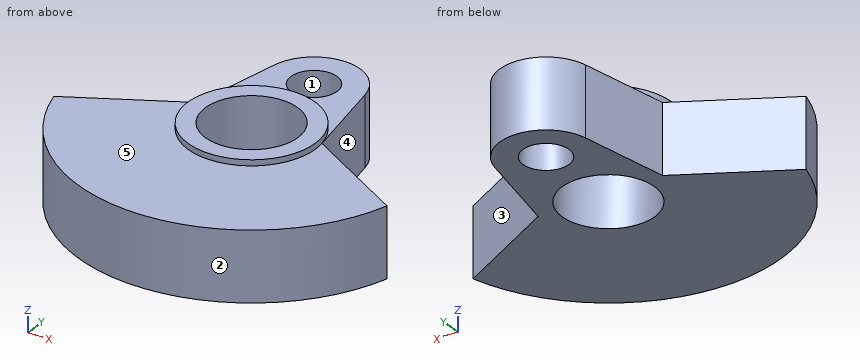
```python
from build123d import *

# Parameters (mm, degrees)
SKETCH1_R           = 2
SKETCH1_R_2         = 4
BOSS_EXTRUDE1_DEPTH = 6
SKETCH2_R           = 5.5
BOSS_EXTRUDE2_DEPTH = 0.5
CUT_EXTRUDE1_START  = -10.5
SKETCH3_R           = 4
CUT_EXTRUDE1_DEPTH  = 10.5


with BuildPart() as part:
    # Sketch1 → Boss-Extrude1 (new body)
    with BuildSketch(Plane.XY):
        with BuildLine():
            Line((-5.402455316, -6.96875), (-3.929058411, 0.75))
            ThreePointArc((-3.929058411, 0.75), (0, 4), (3.929058411, 0.75))
            Line((3.929058411, 0.75), (5.402455316, -6.96875))
            Line((5.402455316, -6.96875), (14.456832295, -12))
            ThreePointArc((14.456832295, -12), (0, -23), (-14.456832295, -12))
            Line((-14.456832295, -12), (-5.402455316, -6.96875))
        make_face()
        Circle(SKETCH1_R, mode=Mode.SUBTRACT)
        with Locations((0, -8)):
            Circle(SKETCH1_R_2, mode=Mode.SUBTRACT)
    extrude(amount=BOSS_EXTRUDE1_DEPTH)

    # Sketch2 → Boss-Extrude2 (add)
    with BuildSketch(Plane.XY.offset(6)):
        with Locations(Location((0, -8, 0), (0, 0, 169.193077125))):
            Circle(SKETCH2_R)
    extrude(amount=BOSS_EXTRUDE2_DEPTH)

    # Sketch3 → Cut-Extrude1 (cut)
    with BuildSketch(Plane.XY.offset(6.5).offset(CUT_EXTRUDE1_START)):
        with Locations((0, -8)):
            Circle(SKETCH3_R)
    extrude(amount=CUT_EXTRUDE1_DEPTH, mode=Mode.SUBTRACT)


solid = part.part
```
Check sheet for the modelled part. Datum: model origin and axes. Units: mm. Face numbers are marked on the shaded views. A direction names the side the tool comes from. Give positions to 0.01 mm unless a question says otherwise; leave off trailing zeros. Order: outer loops, then holes, each group sorted by start corner. A loop starts at its lowest first (then second) coordinate and runs counter-clockwise, first axis right, second up. Notation, with made-up numbers: M 55.5,-14.75 L 75.5,-14.75 A9 ccw 75.5,-6.75 Z; hole C -2,22 d8. An arc over 180 degrees is marked long. Answer in a Markdown table with one row per item.
1) Cross-section at C-C, the plane y = -0.5. Enter the section's corners in (x, z).
Filled sheet:
| item | result |
|---|---|
| outline | M -4.17,0 L -1.94,0 L -1.94,6 L -4.17,6 Z; M 1.94,0 L 4.17,0 L 4.17,6 L 1.94,6 Z |
2) Cross-section at A-A, the plane z = 5. Enter the section's corners in (x, y), plus the area to 3 significant figures.
Filled sheet:
| item | result |
|---|---|
| outline | M -14.46,-12 A15 ccw 14.46,-12 L 5.4,-6.97 L 3.93,0.75 A4 ccw -3.93,0.75 L -5.4,-6.97 Z; hole C 0,-8 d8; hole C 0,0 d4 |
| area | 363 mm2 |
3) Access from +Z, -Z, +X, -X, +Y, -Y to the whole of each face (thin tool, end or side, straight path). Record for the marked faces 4 and 5.
Filled sheet:
| item | result |
|---|---|
| face 4 | +Z, -Z, +X, +Y |
| face 5 | +Z, -Y |
4) Cross-section at B-B, the plane x = 0. Enter the section's corners in (y, z), plus the area to 3 significant figures.
Filled sheet:
| item | result |
|---|---|
| outline | M -23,0 L -12,0 L -12,6.5 L -13.5,6.5 L -13.5,6 L -23,6 Z; M -4,0 L -2,0 L -2,6 L -2.5,6 L -2.5,6.5 L -4,6.5 Z; M 2,0 L 4,0 L 4,6 L 2,6 Z |
| area | 91.5 mm2 |
5) Gauge pin test, flat ends, axial feed: P1, Ø8.5, axis at x = -2, y = -1.5, coming from the +Z side; P2, Ø3, axis at x = -4, z = 3, coming from the -Y side; P3, Ø3, axis at y = -7, z = 5, coming from the +X side; P4, Ø1.5, axis at y = -20, z = 1.5, coming from the +X side. Record the tip position at first contact, or that the pin passes through.
Filled sheet:
| item | result |
|---|---|
| P1 | stops at z = 6.5 |
| P2 | stops at y = -22.79 |
| P3 | stops at x = 8.16 |
| P4 | stops at x = 9.92 |
6) Cross-section at D-D, the plane y = -8. Enter the section's corners in (x, z), plus the area to 3 significant figures.
Filled sheet:
| item | result |
|---|---|
| outline | M -7.26,0 L -4,0 L -4,6.5 L -5.5,6.5 L -5.5,6 L -7.26,6 Z; M 4,0 L 7.26,0 L 7.26,6 L 5.5,6 L 5.5,6.5 L 4,6.5 Z |
| area | 40.6 mm2 |
7) Release check for a two-part mould opening along Y. For the marked faces 1, 2 and 3 record: +Y half, -Y half, draft (parallel to the pull), parting line (faces both ways), or undercut.
Filled sheet:
| item | result |
|---|---|
| face 1 | undercut |
| face 2 | -Y half |
| face 3 | +Y half |
8) Thickness scan on L1, parallel to Y at x = 0, z = 4; L2, parallel to Z at x = 2.5, y = -14; L3, parallel to X at y = -8.5, z = 0.5. Record the ranges inside material, lowest first. Write a range as [from, to].
Filled sheet:
| item | result |
|---|---|
| L1 | y = [-23, -12], [-4, -2], [2, 4] |
| L2 | z = [0, 6] |
| L3 | x = [-8.16, -3.97], [3.97, 8.16] |
